from build123d import *

# Parameters (mm, degrees)
F1_DEPTH   = 35
F3_D       = 2.7
F5_DEPTH   = 1
F6_DEPTH   = 1
F9_D       = 2.7
F9_ON_F7_D = 2.7
F8_W       = 1.6217698948
F8_H       = 2.85
F10_DEPTH  = 1
F11_DEPTH  = 1


# Not quite as in the source:
# - a feature names something its author has since deleted; it is built from what else it names


with BuildPart() as f1:
    # F0 (on Top) → F1 (new body)
    with BuildSketch(Plane.XY):
        with BuildLine():
            Line((-21.3074208284, -25.7097307226), (-27.8221394541, -25.7097307226))
            ThreePointArc((-27.8221394541, -25.7097307226), (-41.1900200037, -21.1492925546), (-42.5323706273, -35.2097307226))
            Line((-42.5323706273, -35.2097307226), (-68.0612095771, -35.2097307226))
            ThreePointArc((-68.0612095771, -35.2097307226), (-71.4714049121, -19.3897012131), (-86.3697267271, -25.7097307226))
            Line((-86.3697267271, -25.7097307226), (-92.8074208284, -25.7097307226))
            Line((-92.8074208284, -25.7097307226), (-92.8074208284, -28.2097307226))
            Line((-92.8074208284, -28.2097307226), (-83.7907356019, -28.2097307226))
            ThreePointArc((-83.7907356019, -28.2097307226), (-68.8074208284, -28.7097307226), (-83.7907356019, -29.2097307226))
            Line((-83.7907356019, -29.2097307226), (-92.8074208284, -29.2097307226))
            Line((-92.8074208284, -29.2097307226), (-92.8074208284, -31.7097307226))
            Line((-92.8074208284, -31.7097307226), (-86.3697267271, -31.7097307226))
            ThreePointArc((-86.3697267271, -31.7097307226), (-85.5676654464, -33.6592629847), (-84.3923404334, -35.4092885424))
            Line((-84.3923404334, -35.4092885424), (-84.3923404334, -36.2097307226))
            ThreePointArc((-84.3923404334, -36.2097307226), (-83.5136607769, -38.3310510662), (-81.3923404334, -39.2097307226))
            Line((-81.3923404334, -39.2097307226), (-32.3990289542, -39.2097307226))
            ThreePointArc((-32.3990289542, -39.2097307226), (-30.9848153918, -38.623944285), (-30.3990289542, -37.2097307226))
            Line((-30.3990289542, -37.2097307226), (-30.3990289542, -35.4987590376))
            ThreePointArc((-30.3990289542, -35.4987590376), (-28.8654021984, -33.7709913079), (-27.8221394541, -31.7097307226))
            Line((-27.8221394541, -31.7097307226), (-21.3074208284, -31.7097307226))
            Line((-21.3074208284, -31.7097307226), (-21.3074208284, -29.2097307226))
            Line((-21.3074208284, -29.2097307226), (-30.3282904568, -29.2097307226))
            ThreePointArc((-30.3282904568, -29.2097307226), (-42.3074208284, -28.7097307226), (-30.3282904568, -28.2097307226))
            Line((-30.3282904568, -28.2097307226), (-21.3074208284, -28.2097307226))
            Line((-21.3074208284, -28.2097307226), (-21.3074208284, -25.7097307226))
        make_face()
    extrude(amount=F1_DEPTH)

    # F3 (through all)
    with Locations(Plane.XZ.offset(39.2097307226)):
        with Locations((-63.8074208284, 30), (-48.80741708, 30), (-48.80741708, 5), (-63.8074208284, 5)):
            Hole(F3_D / 2)

    # F4 (on face) → F5 (cut)
    with BuildSketch(Plane(origin=(0, -35.2097307226, 0), x_dir=(-1, 0, 0), z_dir=(0, 1, 0))):
        Polygon((50.4817328606, 27.1), (52.1560486413, 30), (50.4817328606, 32.9), (47.1331012993, 32.9), (45.4587855187, 30), (47.1331012993, 27.1), align=None)
        Polygon((62.1331050477, 32.9), (60.4587892671, 30), (62.1331050477, 27.1), (65.481736609, 27.1), (67.1560523897, 30), (65.481736609, 32.9), align=None)
        Polygon((52.1560486413, 5), (50.4817328606, 7.9), (47.1331012993, 7.9), (45.4587855187, 5), (47.1331012993, 2.1), (50.4817328606, 2.1), align=None)
        Polygon((62.1331050477, 2.1), (65.481736609, 2.1), (67.1560523897, 5), (65.481736609, 7.9), (62.1331050477, 7.9), (60.4587892671, 5), align=None)
    extrude(amount=-F5_DEPTH, mode=Mode.SUBTRACT)

    # F6 (add): a face of the model
    f6_faces = [f1.faces().sort_by_distance(p)[0] for p in [
        (-55.1452142049, -35.2097307226, 17.5),
    ]]
    extrude(f6_faces, amount=F6_DEPTH)

    # F9 (through all)
    with Locations(Plane(origin=(0, -25.7097307226, 0), x_dir=(-1, 0, 0), z_dir=(0, 1, 0))):
        with Locations((24.5647801412, 26), (24.5647801412, 9)):
            Hole(F9_D / 2)

    # F9 on F7 (through all)
    with Locations(Plane(origin=(0, -25.7097307226, 0), x_dir=(-1, 0, 0), z_dir=(0, 1, 0))):
        with Locations((89.5885737777, 9), (89.5885737777, 26)):
            Hole(F9_ON_F7_D / 2)

    # F8 (on face) → F10 (cut)
    with BuildSketch(Plane(origin=(0, -25.7097307226, 0), x_dir=(-1, 0, 0), z_dir=(0, 1, 0))):
        Polygon((26.2102284084, 28.85), (24.5647801412, 28.85), (24.5647801412, 26), (26.1865500361, 26), (26.1865500361, 23.15), (26.2102284084, 23.15), (27.8556766756, 26), align=None)
        Polygon((24.5647801412, 26), (24.5647801412, 28.85), (22.919331874, 28.85), (21.2738836069, 26), (22.919331874, 23.15), (24.5647801412, 23.15), align=None)
        with Locations((25.3756650887, 10.425)):
            Rectangle(F8_W, F8_H)
        Polygon((24.5647801412, 9), (24.5647801412, 11.85), (22.919331874, 11.85), (21.2738836069, 9), (22.919331874, 6.15), (24.5647801412, 6.15), align=None)
        with Locations((25.3756650887, 24.575)):
            Rectangle(F8_W, F8_H)
        Polygon((26.1865500361, 9), (24.5647801412, 9), (24.5647801412, 6.15), (26.2102284084, 6.15), (27.8556766756, 9), (26.2102284084, 11.85), (26.1865500361, 11.85), align=None)
    extrude(amount=-F10_DEPTH, mode=Mode.SUBTRACT)

    # F7 (on face) → F11 (cut)
    with BuildSketch(Plane(origin=(0, -25.7097307226, 0), x_dir=(-1, 0, 0), z_dir=(0, 1, 0))):
        Polygon((91.2340220449, 6.15), (92.8794703121, 9), (91.2340220449, 11.85), (87.9431255105, 11.85), (86.2976772433, 9), (87.9431255105, 6.15), align=None)
        Polygon((92.8794703121, 26), (91.2340220449, 28.85), (87.9431255105, 28.85), (86.2976772433, 26), (87.9431255105, 23.15), (91.2340220449, 23.15), align=None)
    extrude(amount=-F11_DEPTH, mode=Mode.SUBTRACT)


solid = f1.part
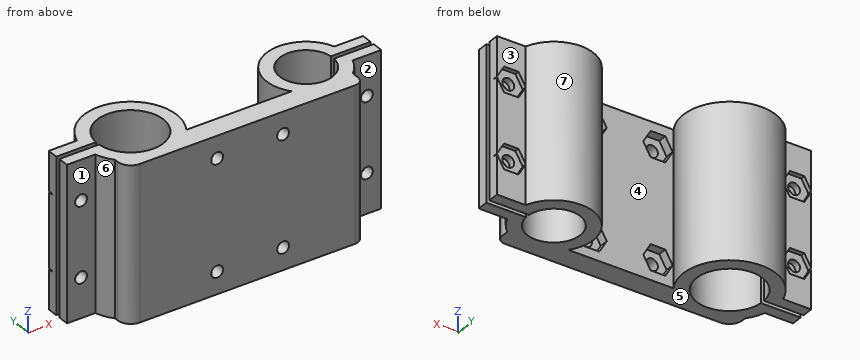
Geometry check sheet. Reference: the model listing, model coordinates, mm. Face numbers are marked on the shaded views. A direction names the side the tool comes from. Round coordinates to 2 decimals unless told otherwise and drop trailing zeros. Write each loop counter-clockwise with the first axis right and the second up, starting at its lowest first coordinate (ties: lowest second). Pieces come first, ordered by that corner, then holes.
Item 1: Section check B-B (z = 21). Record the boundary of the cut face in (x, y), plus the area to 3 significant figures.
Determined:
outline: (-92.81, -31.71) - (-86.37, -31.71) arc R10.5 ccw to (-84.39, -35.41) - (-84.39, -36.21) arc R3 ccw to (-81.39, -39.21) - (-32.4, -39.21) arc R2 ccw to (-30.4, -37.21) - (-30.4, -35.5) arc R9 ccw to (-27.82, -31.71) - (-21.31, -31.71) - (-21.31, -29.21) - (-30.33, -29.21) arc R6 cw (long way) to (-30.33, -28.21) - (-21.31, -28.21) - (-21.31, -25.71) - (-27.82, -25.71) arc R9 ccw (long way) to (-43.43, -34.21) - (-67.36, -34.21) arc R10.5 ccw (long way) to (-86.37, -25.71) - (-92.81, -25.71) - (-92.81, -28.21) - (-83.79, -28.21) arc R7.5 cw (long way) to (-83.79, -29.21) - (-92.81, -29.21) - close
area: 537 mm2
Item 2: Section check A-A (y = -30). Record the boundary of the cut face in (x, z), plus the area to 3 significant figures.
Determined:
outline: (-92.81, 0) - (-83.7, 0) - (-83.7, 35) - (-92.81, 35) - close; (-68.92, 0) - (-65.89, 0) - (-65.89, 35) - (-68.92, 35) - close; (-45.21, 0) - (-42.17, 0) - (-42.17, 35) - (-45.21, 35) - close; (-30.45, 0) - (-21.31, 0) - (-21.31, 35) - (-30.45, 35) - close; hole circle Ø2.7 at (-89.59, 9); hole circle Ø2.7 at (-89.59, 26); hole circle Ø2.7 at (-24.56, 9); hole circle Ø2.7 at (-24.56, 26)
area: 829 mm2
Item 3: Section check D-D (x = -37.5). Record the boundary of the cut face in (y, z), plus the area to 3 significant figures.
Determined:
outline: (-39.21, 0) - (-34.59, 0) - (-34.59, 35) - (-39.21, 35) - close; (-22.83, 0) - (-19.79, 0) - (-19.79, 35) - (-22.83, 35) - close
area: 268 mm2
Item 4: Section check C-C (x = -77.5). Record the boundary of the cut face in (y, z).
Determined:
outline: (-39.21, 0) - (-36.11, 0) - (-36.11, 35) - (-39.21, 35) - close; (-21.31, 0) - (-18.28, 0) - (-18.28, 35) - (-21.31, 35) - close
Item 5: Access from +Z, -Z, +X, -X, +Y, -Y to the whole of each face (thin tool, end or side, straight path). Record for the marked faces 1, 2 and 3.
Determined:
face 1: +Z, -Z, -X, -Y
face 2: +Z, -Z, +X, -Y
face 3: +Z, -Z, +X, +Y
Item 6: Material ranges on line 1 along Y through (x, z) = (-88, 33.5); line 2 along X through (y, z) = (-26.5, 6); line 3 along X through (y, z) = (-26.75, 22), recorded low to high.
Determined:
line 1: y = -31.71 to -29.21, -28.21 to -25.71
line 2: x = -92.81 to -83.47, -69.14 to -66.04, -45.03 to -41.89, -30.73 to -21.31
line 3: x = -92.81 to -83.55, -69.07 to -65.99, -45.09 to -41.98, -30.64 to -21.31
Item 7: Go/stop test with flat-tipped pins: pin 1 Ø0.5 at (y, z) = (-36.5, 13) entering from +X; pin 2 Ø5 at (x, z) = (-23.5, 18) entering from -Y; pin 3 Ø3 at (x, z) = (-49.5, 4) entering from +Y. Record where each tip stops, or that it passes through.
Determined:
pin 1: stops at x = -30.4
pin 2: stops at y = -31.71
pin 3: stops at y = -36.21
Item 8: Mould release check, pull along X, two halves, no side actions. Record for the marked faces 4, 5, 6 and 7: +X half, -X half, draft (parallel to the pull), parting line (faces both ways), or undercut.
Determined:
face 4: undercut
face 5: draft
face 6: -X half
face 7: undercut
